Autodesk Fusion 360 part; units mm, degrees
sketch "plate-2025-06-26T05_56_28.958Z" plane through (0, 0, 0) normal (0, 0, 1) x (1, 0, 0)
  line L0 (22.075, -2.525) -> (35.075, -2.525)
  line L1 (22.075, -16.525) -> (35.075, -16.525)
  line L2 (21.575, -3.025) -> (21.575, -16.025)
  line L3 (35.575, -3.025) -> (35.575, -16.025)
  arc A0 (22.075, -2.525) -> (21.575, -3.025) centre (22.075, -3.025) ccw
  arc A1 (35.575, -3.025) -> (35.075, -2.525) centre (35.075, -3.025) ccw
  arc A2 (21.575, -16.025) -> (22.075, -16.525) centre (22.075, -16.025) ccw
  arc A3 (35.075, -16.525) -> (35.575, -16.025) centre (35.075, -16.025) ccw
  line L4 (41.125, -2.525) -> (54.125, -2.525)
  line L5 (41.125, -16.525) -> (54.125, -16.525)
  line L6 (40.625, -3.025) -> (40.625, -16.025)
  line L7 (54.625, -3.025) -> (54.625, -16.025)
  arc A4 (41.125, -2.525) -> (40.625, -3.025) centre (41.125, -3.025) ccw
  arc A5 (54.625, -3.025) -> (54.125, -2.525) centre (54.125, -3.025) ccw
  arc A6 (40.625, -16.025) -> (41.125, -16.525) centre (41.125, -16.025) ccw
  arc A7 (54.125, -16.525) -> (54.625, -16.025) centre (54.125, -16.025) ccw
  line L8 (60.175, -2.525) -> (73.175, -2.525)
  line L9 (60.175, -16.525) -> (73.175, -16.525)
  line L10 (59.675, -3.025) -> (59.675, -16.025)
  line L11 (73.675, -3.025) -> (73.675, -16.025)
  arc A8 (60.175, -2.525) -> (59.675, -3.025) centre (60.175, -3.025) ccw
  arc A9 (73.675, -3.025) -> (73.175, -2.525) centre (73.175, -3.025) ccw
  arc A10 (59.675, -16.025) -> (60.175, -16.525) centre (60.175, -16.025) ccw
  arc A11 (73.175, -16.525) -> (73.675, -16.025) centre (73.175, -16.025) ccw
  line L12 (138.92, -30.97) -> (-14.8, -30.97)
  line L13 (-14.8, -30.97) -> (-14.8, 11.89)
  line L14 (-14.8, 11.89) -> (138.92, 11.89)
  line L15 (138.92, 11.89) -> (138.92, -30.97)
  line L16 (128.92, 1.89) -> (-4.8, 1.89)
  line L17 (-4.8, 1.89) -> (-4.8, -20.97)
  line L18 (-4.8, -20.97) -> (128.92, -20.97)
  line L19 (128.92, -20.97) -> (128.92, 1.89)
  circle A12 centre (133.92, 6.89) radius 1.7
  circle A13 centre (133.92, -25.97) radius 1.7
  circle A14 centre (-9.8, -25.97) radius 1.7
  circle A15 centre (-9.8, 6.89) radius 1.7
  arc A16 (54.625, -3.025) -> (54.125, -2.525) centre (54.125, -3.025) ccw
  line L20 (21.575, -3.025) -> (21.575, -16.025)
  arc A17 (60.175, -2.525) -> (59.675, -3.025) centre (60.175, -3.025) ccw
  arc A18 (54.125, -16.525) -> (54.625, -16.025) centre (54.125, -16.025) ccw
  line L21 (40.625, -3.025) -> (40.625, -16.025)
  line L22 (35.575, -3.025) -> (35.575, -16.025)
  line L23 (59.675, -3.025) -> (59.675, -16.025)
  line L24 (22.075, -16.525) -> (35.075, -16.525)
  line L25 (41.125, -16.525) -> (54.125, -16.525)
  arc A19 (41.125, -2.525) -> (40.625, -3.025) centre (41.125, -3.025) ccw
  line L26 (60.175, -2.525) -> (73.175, -2.525)
  line L27 (54.625, -3.025) -> (54.625, -16.025)
  arc A20 (22.075, -2.525) -> (21.575, -3.025) centre (22.075, -3.025) ccw
  arc A21 (73.675, -3.025) -> (73.175, -2.525) centre (73.175, -3.025) ccw
  line L28 (73.675, -3.025) -> (73.675, -16.025)
  arc A22 (35.075, -16.525) -> (35.575, -16.025) centre (35.075, -16.025) ccw
  arc A23 (35.575, -3.025) -> (35.075, -2.525) centre (35.075, -3.025) ccw
  arc A24 (21.575, -16.025) -> (22.075, -16.525) centre (22.075, -16.025) ccw
  line L29 (60.175, -16.525) -> (73.175, -16.525)
  arc A25 (59.675, -16.025) -> (60.175, -16.525) centre (60.175, -16.025) ccw
  arc A26 (40.625, -16.025) -> (41.125, -16.525) centre (41.125, -16.025) ccw
  line L30 (41.125, -2.525) -> (54.125, -2.525)
  arc A27 (73.175, -16.525) -> (73.675, -16.025) centre (73.175, -16.025) ccw
  line L31 (22.075, -2.525) -> (35.075, -2.525)
  line L32 (79.225, -2.525) -> (92.225, -2.525)
  line L33 (98.275, -2.525) -> (111.275, -2.525)
  arc A28 (111.275, -16.525) -> (111.775, -16.025) centre (111.275, -16.025) ccw
  line L34 (111.775, -3.025) -> (111.775, -16.025)
  arc A29 (111.775, -3.025) -> (111.275, -2.525) centre (111.275, -3.025) ccw
  arc A30 (111.275, -16.525) -> (111.775, -16.025) centre (111.275, -16.025) ccw
  line L35 (79.225, -16.525) -> (92.225, -16.525)
  line L36 (98.275, -2.525) -> (111.275, -2.525)
  line L37 (98.275, -16.525) -> (111.275, -16.525)
  arc A31 (79.225, -2.525) -> (78.725, -3.025) centre (79.225, -3.025) ccw
  arc A32 (92.225, -16.525) -> (92.725, -16.025) centre (92.225, -16.025) ccw
  arc A33 (111.775, -3.025) -> (111.275, -2.525) centre (111.275, -3.025) ccw
  arc A34 (97.775, -16.025) -> (98.275, -16.525) centre (98.275, -16.025) ccw
  arc A35 (98.275, -2.525) -> (97.775, -3.025) centre (98.275, -3.025) ccw
  arc A36 (92.225, -16.525) -> (92.725, -16.025) centre (92.225, -16.025) ccw
  line L38 (111.775, -3.025) -> (111.775, -16.025)
  line L39 (97.775, -3.025) -> (97.775, -16.025)
  line L40 (98.275, -16.525) -> (111.275, -16.525)
  arc A37 (79.225, -2.525) -> (78.725, -3.025) centre (79.225, -3.025) ccw
  line L41 (92.725, -3.025) -> (92.725, -16.025)
  arc A38 (92.725, -3.025) -> (92.225, -2.525) centre (92.225, -3.025) ccw
  line L42 (78.725, -3.025) -> (78.725, -16.025)
  line L43 (97.775, -3.025) -> (97.775, -16.025)
  arc A39 (78.725, -16.025) -> (79.225, -16.525) centre (79.225, -16.025) ccw
  line L44 (92.725, -3.025) -> (92.725, -16.025)
  line L45 (79.225, -2.525) -> (92.225, -2.525)
  arc A40 (97.775, -16.025) -> (98.275, -16.525) centre (98.275, -16.025) ccw
  arc A41 (92.725, -3.025) -> (92.225, -2.525) centre (92.225, -3.025) ccw
  arc A42 (98.275, -2.525) -> (97.775, -3.025) centre (98.275, -3.025) ccw
  line L46 (78.725, -3.025) -> (78.725, -16.025)
  arc A43 (78.725, -16.025) -> (79.225, -16.525) centre (79.225, -16.025) ccw
  line L47 (79.225, -16.525) -> (92.225, -16.525)
  dimension "d1" = 153.72
  dimension "d2" = 42.86
  dimension "d9" = 10
  dimension "d11" = 5.05
  dimension "d12" = 5.05
  dimension "d13" = 3.4
  dimension "d14" = 3.4
  dimension "d15" = 3.4
  dimension "d16" = 3.4
  dimension "d17" = 5
  dimension "d18" = 5
  dimension "d19" = 5
  dimension "d20" = 5
  dimension "d21" = 5
  dimension "d22" = 5
  dimension "d23" = 5
  dimension "d24" = 5
  dimension "d29" = 10
  dimension "d30" = 10
  dimension "d31" = 10
  dimension "d32" = 26.375
  dimension "d33" = 5.05
  dimension "d34" = 5.05
  dimension "d35" = 5.05
  dimension "d36" = 5.05
extrude "Extrude1" add sketch "plate-2025-06-26T05_56_28.958Z" along normal blind 1.5 contours L12 L13 L14 L15 | L16 L17 L18 L19
fillet "Fillet1" radius 5 4 edges at (138.92, -30.97, 0.75) (138.92, 11.89, 0.75) (-14.8, -30.97, 0.75) (-14.8, 11.89, 0.75)
equation "d1 = 115.620 mm + 38.1 mm"
The listing builds one solid part. Answer for the finished solid, in the listing's coordinates (mm). Round coordinates to 2 decimals unless told otherwise and drop trailing zeros. Write each loop counter-clockwise with the first axis right and the second up, starting at its lowest first coordinate (ties: lowest second). Pieces come first, ordered by that corner, then holes. Notation, with made-up numbers: (-6.5, 67.5) -> (18.5, 67.5) arc R19 cw to (18.5, 71.5) -> close; hole circle Ø7 at (44.5, -14.75). An arc over 180 degrees is marked (long way). Write item = value, one per line.
1) Section B-B on z = 0.5 is taken. Give the number of separate pieces and of enclosed holes in the cut face, plus the area to 3 significant figures.
Check values:
separate_pieces = 1
enclosed_holes = 9
area = 5,550 mm²
2) Section A-A on y = -12 is taken. Write down the section's boundary in (x, z) (3 decimals), plus the area to 3 significant figures.
Check values:
outline = (-14.8, 0) -> (21.575, 0) -> (21.575, 1.5) -> (-14.8, 1.5) -> close; (35.575, 0) -> (40.625, 0) -> (40.625, 1.5) -> (35.575, 1.5) -> close; (54.625, 0) -> (59.675, 0) -> (59.675, 1.5) -> (54.625, 1.5) -> close; (73.675, 0) -> (78.725, 0) -> (78.725, 1.5) -> (73.675, 1.5) -> close; (92.725, 0) -> (97.775, 0) -> (97.775, 1.5) -> (92.725, 1.5) -> close; (111.775, 0) -> (138.92, 0) -> (138.92, 1.5) -> (111.775, 1.5) -> close
area = 126 mm²
3) Straight lines are drawn through the part: line 1 along X through (y, z) = (-12, 0.95) (3 decimals); line 2 along Y through (x, z) = (133.92, 1.1); line 3 along Y through (x, z) = (64, 1.35) (3 decimals). For each, find the intervals that lie inside material, in ascending order. Write a range as [from, to].
Check values:
line_1 = [-14.8, 21.575], [35.575, 40.625], [54.625, 59.675], [73.675, 78.725], [92.725, 97.775], [111.775, 138.92]
line_2 = [-30.97, -27.67], [-24.27, 5.19], [8.59, 11.89]
line_3 = [-30.97, -16.525], [-2.525, 11.89]
4) For a pull along Y with two mould halves and no side action, classify faces 1 (the flat face through (61, 0, 0)), 2 (the cylindrical face through (134.834, 5.457, 0.74)), 3 (the cylindrical face through (-13.3, 10.46, 0.76)) as released by +Y, released by -Y, zero draft, split by the parting line, or undercut.
Check values:
face_1 = zero draft
face_2 = undercut
face_3 = released by +Y
